```python
from build123d import *

# Parameters (mm, degrees)
SKETCH_1_R      = 1.55
SKETCH_1_W      = 10
SKETCH_1_H      = 6.1
EXTRUDE_1_DEPTH = 6


with BuildPart() as part:
    # Эскиз1 → Бобышка-Вытянуть1 (new body)
    with BuildSketch(Plane(origin=(0, 0, 0), x_dir=(1, 0, 0), z_dir=(0, 1, 0))):
        Polygon((10.144022003, 31.870182818), (9.894022003, 25.870182818), (-15.605977997, 25.870182818), (-15.855977997, 31.870182818), (-25.855977997, 31.870182818), (-26.105977997, 25.870182818), (-31.305977997, 25.870182818), (-31.305977997, 19.070182818), (-30.105977997, 19.070182818), (-30.105977997, 16.870182818), (-31.305977997, 16.870182818), (-31.305977997, 15.370182818), (-34.405977997, 15.370182818), (-34.405977997, 16.870182818), (-35.605977997, 16.870182818), (-35.605977997, 19.070182818), (-34.405977997, 19.070182818), (-34.405977997, 25.870182818), (-39.605977997, 25.870182818), (-39.855977997, 31.870182818), (-49.855977997, 31.870182818), (-50.105977997, 25.870182818), (-83.355977997, 25.870182818), (-83.355977997, 21.420182818), (-78.555977997, 21.420182818), (-78.555977997, 22.620182818), (-76.355977997, 22.620182818), (-76.355977997, 21.420182818), (-74.855977997, 21.420182818), (-74.855977997, 18.320182818), (-76.355977997, 18.320182818), (-76.355977997, 17.120182818), (-78.555977997, 17.120182818), (-78.555977997, 18.320182818), (-83.355977997, 18.320182818), (-83.355977997, 7.370182818), (-101.355977997, 7.370182818), (-101.355977997, -7.629817182), (-83.355977997, -7.629817182), (-83.355977997, -18.579817182), (-78.555977997, -18.579817182), (-78.555977997, -17.379817182), (-76.355977997, -17.379817182), (-76.355977997, -18.579817182), (-74.855977997, -18.579817182), (-74.855977997, -21.679817182), (-76.355977997, -21.679817182), (-76.355977997, -22.879817182), (-78.555977997, -22.879817182), (-78.555977997, -21.679817182), (-83.355977997, -21.679817182), (-83.355977997, -26.129817182), (-50.105977997, -26.129817182), (-49.855977997, -32.129817182), (-39.855977997, -32.129817182), (-39.605977997, -26.129817182), (-34.405977997, -26.129817182), (-34.405977997, -19.329817182), (-35.605977997, -19.329817182), (-35.605977997, -17.129817182), (-34.405977997, -17.129817182), (-34.405977997, -15.629817182), (-31.305977997, -15.629817182), (-31.305977997, -17.129817182), (-30.105977997, -17.129817182), (-30.105977997, -19.329817182), (-31.305977997, -19.329817182), (-31.305977997, -26.129817182), (-26.105977997, -26.129817182), (-25.855977997, -32.129817182), (-15.855977997, -32.129817182), (-15.605977997, -26.129817182), (9.894022003, -26.129817182), (10.144022003, -32.129817182), (20.144022003, -32.129817182), (20.394022003, -26.129817182), (25.594022003, -26.129817182), (25.594022003, -19.329817182), (24.394022003, -19.329817182), (24.394022003, -17.129817182), (25.594022003, -17.129817182), (25.594022003, -15.629817182), (28.694022003, -15.629817182), (28.694022003, -17.129817182), (29.894022003, -17.129817182), (29.894022003, -19.329817182), (28.694022003, -19.329817182), (28.694022003, -26.129817182), (33.894022003, -26.129817182), (34.144022003, -32.129817182), (44.144022003, -32.129817182), (44.394022003, -26.129817182), (77.644022003, -26.129817182), (77.644022003, -21.679817182), (72.844022003, -21.679817182), (72.844022003, -22.879817182), (70.644022003, -22.879817182), (70.644022003, -21.679817182), (69.144022003, -21.679817182), (69.144022003, -18.579817182), (70.644022003, -18.579817182), (70.644022003, -17.379817182), (72.844022003, -17.379817182), (72.844022003, -18.579817182), (77.644022003, -18.579817182), (77.644022003, -7.629817182), (95.644022003, -7.629817182), (95.644022003, 7.370182818), (77.644022003, 7.370182818), (77.644022003, 18.320182818), (72.844022003, 18.320182818), (72.844022003, 17.120182818), (70.644022003, 17.120182818), (70.644022003, 18.320182818), (69.144022003, 18.320182818), (69.144022003, 21.420182818), (70.644022003, 21.420182818), (70.644022003, 22.620182818), (72.844022003, 22.620182818), (72.844022003, 21.420182818), (77.644022003, 21.420182818), (77.644022003, 25.870182818), (44.394022003, 25.870182818), (44.144022003, 31.870182818), (34.144022003, 31.870182818), (33.894022003, 25.870182818), (28.694022003, 25.870182818), (28.694022003, 19.070182818), (29.894022003, 19.070182818), (29.894022003, 16.870182818), (28.694022003, 16.870182818), (28.694022003, 15.370182818), (25.594022003, 15.370182818), (25.594022003, 16.870182818), (24.394022003, 16.870182818), (24.394022003, 19.070182818), (25.594022003, 19.070182818), (25.594022003, 25.870182818), (20.394022003, 25.870182818), (20.144022003, 31.870182818), align=None)
        with Locations((-32.855977997, -0.129817182)):
            Circle(SKETCH_1_R, mode=Mode.SUBTRACT)
        with Locations((27.144022003, -0.129817182)):
            Circle(SKETCH_1_R, mode=Mode.SUBTRACT)
        with Locations((-20.855977997, -0.129817182)):
            Rectangle(SKETCH_1_W, SKETCH_1_H, mode=Mode.SUBTRACT)
        with Locations((-44.855977997, -0.129817182)):
            Rectangle(SKETCH_1_W, SKETCH_1_H, mode=Mode.SUBTRACT)
        with Locations((15.144022003, -0.129817182)):
            Rectangle(SKETCH_1_W, SKETCH_1_H, mode=Mode.SUBTRACT)
        with Locations((39.144022003, -0.129817182)):
            Rectangle(SKETCH_1_W, SKETCH_1_H, mode=Mode.SUBTRACT)
    extrude(amount=EXTRUDE_1_DEPTH)


solid = part.part
```
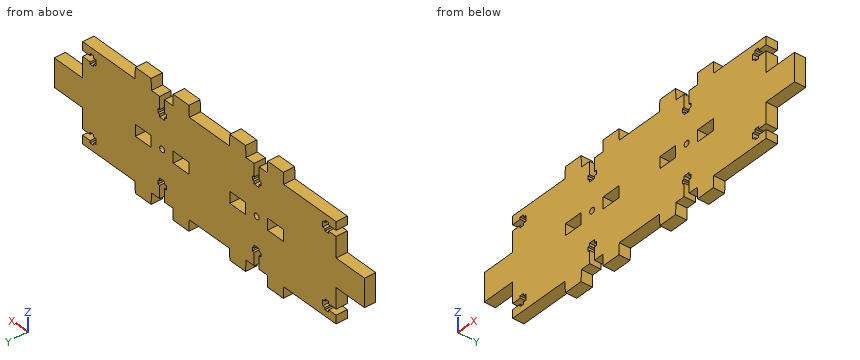
Work out the finished part from the listing and answer in its coordinate system (mm). Coordinates: 2 decimals unless noted, no trailing zeros. Loops run counter-clockwise (first coordinate to the right, second up) from the corner with the lowest first, then second, coordinate; pieces in that order, holes last.
1) Section B-B (z = -12) is taken. Give the vertices of the cut face in (x, y), plus the area to 3 significant figures.
Results:
outline: (-83.36, 0) - (77.64, 0) - (77.64, 6) - (-83.36, 6) - close
area: 966 mm2
2) Section C-C (x = -89) is taken. Give the vertices of the cut face in (y, z), plus the area to 3 significant figures.
Results:
outline: (0, -7.37) - (6, -7.37) - (6, 7.63) - (0, 7.63) - close
area: 90.0 mm2
3) Consider probe 1 along X at (y, z) = (5.45, -19); probe 2 along Z at (x, y) = (-18, 4); probe 3 along X at (y, z) = (4.9, -21). Determine where each line is inside the solid, lowest interval first.
Results:
probe 1: x = -74.86 to -35.61, -30.11 to 24.39, 29.89 to 69.14
probe 2: z = -31.87 to -2.92, 3.18 to 32.13
probe 3: x = -74.86 to -34.41, -31.31 to 25.59, 28.69 to 69.14
4) Flat-ended cylindrical pins translate along their axes: pin 1 (0.7 mm diameter, centred on x = 72, y = 3.5, fed in from +Z); pin 2 (2.5 mm diameter, centred on y = 1.5, z = 18.5, fed in from +X); pin 3 (3 mm diameter, centred on x = -0.5, y = 5, fed in from -Z). Find the tip coordinate at first contact, or state that the pin passes through.
Results:
pin 1: stops at z = 26.13
pin 2: stops at x = 77.64
pin 3: stops at z = -25.87
5) Section D-D (y = 3.1) is taken. Give the number of separate pieces and of enclosed holes in the cut face, plus the area to 3 significant figures.
Results:
separate pieces: 1
enclosed holes: 6
area: 8,870 mm2
6) Section A-A (x = 16) is taken. Give the vertices of the cut face in (y, z), plus the area to 3 significant figures.
Results:
outline: (0, -31.87) - (6, -31.87) - (6, -2.92) - (0, -2.92) - close; (0, 3.18) - (6, 3.18) - (6, 32.13) - (0, 32.13) - close
area: 347 mm2
